from build123d import *

# Parameters (mm, degrees)
SKETCH3_R           = 15
BOSS_EXTRUDE1_DEPTH = 20
SKETCH4_R           = 2.5
CUT_EXTRUDE1_DEPTH  = 30.154759474
CUT_EXTRUDE2_DEPTH  = 4.5
SKETCH7_W           = 9
SKETCH7_H           = 4.5
CUT_EXTRUDE3_DEPTH  = 30.154759474
BOSS_EXTRUDE3_DEPTH = 10
SKETCH9_R           = 2.5
CUT_EXTRUDE4_DEPTH  = 30
SKETCH12_R          = 23.5
BOSS_EXTRUDE6_DEPTH = 75
SKETCH13_R          = 19
CUT_EXTRUDE6_DEPTH  = 143.195288401
SKETCH14_R          = 19
BOSS_EXTRUDE7_DEPTH = 5
SKETCH15_R          = 1.5
SKETCH15_R_2        = 2.5
CUT_EXTRUDE8_DEPTH  = 5


with BuildPart() as part:
    # Sketch3 → Boss-Extrude1 (new body)
    with BuildSketch(Plane(origin=(0, 0, 0), x_dir=(1, 0, 0), z_dir=(0, 1, 0))):
        with Locations(Location((0, 0, 0), (0, 0, 270))):
            Circle(SKETCH3_R)
    extrude(amount=-BOSS_EXTRUDE1_DEPTH)

    # Sketch4 → Cut-Extrude1 (cut, through all)
    with BuildSketch(Plane(origin=(0, 0, 0), x_dir=(1, 0, 0), z_dir=(0, 1, 0))):
        with Locations(Location((0, 0, 0), (0, 0, 270))):
            Circle(SKETCH4_R)
    extrude(amount=-CUT_EXTRUDE1_DEPTH, mode=Mode.SUBTRACT)

    # Sketch6 → Cut-Extrude2 (cut)
    with BuildSketch(Plane(origin=(0, -5, 0), x_dir=(1, 0, 0), z_dir=(0, 1, 0))):
        Polygon((4.5, -2.598076211), (4.5, 2.598076211), (0, 5.196152423), (-4.5, 2.598076211), (-4.5, -2.598076211), (0, -5.196152423), align=None)
    extrude(amount=-CUT_EXTRUDE2_DEPTH, mode=Mode.SUBTRACT)

    # Sketch7 → Cut-Extrude3 (cut, through all)
    with BuildSketch(Plane.XY):
        with Locations((0, -7.25)):
            Rectangle(SKETCH7_W, SKETCH7_H)
    extrude(amount=CUT_EXTRUDE3_DEPTH, mode=Mode.SUBTRACT)

    # Sketch8 → Boss-Extrude3 (add, symmetric)
    with BuildSketch(Plane(origin=(0, 0, 0), x_dir=(0, 0, -1), z_dir=(1, 0, 0))):
        with BuildLine():
            Line((0, 0), (0, -20))
            add(Edge.make_bspline(
                [(0, -20), (27.284263103, -24.07033424), (42.456200025, -63.400009775), (20, -80)],
                knots=[0, 0, 0, 0, 1, 1, 1, 1], degree=3))
            Line((20, -80), (67.5, -80))
            add(Edge.make_bspline(
                [(0, 0), (41.415251378, -8.894775063), (64.240572417, -43.774170089), (67.5, -80)],
                knots=[0, 0, 0, 0, 1, 1, 1, 1], degree=3))
        make_face()
    extrude(amount=BOSS_EXTRUDE3_DEPTH, both=True)

    # Sketch9 → Cut-Extrude4 (cut)
    with BuildSketch(Plane(origin=(0, 0, 0), x_dir=(1, 0, 0), z_dir=(0, 1, 0))):
        with Locations(Location((0, 0, 0), (0, 0, 270))):
            Circle(SKETCH9_R)
    extrude(amount=-CUT_EXTRUDE4_DEPTH, mode=Mode.SUBTRACT)

    # Sketch12 → Boss-Extrude6 (add)
    with BuildSketch(Plane.XY.offset(-10)):
        with Locations((0, -95)):
            Circle(SKETCH12_R)
    extrude(amount=-BOSS_EXTRUDE6_DEPTH)

    # Sketch13 → Cut-Extrude6 (cut, through all)
    with BuildSketch(Plane.XY.offset(-10)):
        with Locations((0, -95)):
            Circle(SKETCH13_R)
    extrude(amount=-CUT_EXTRUDE6_DEPTH, mode=Mode.SUBTRACT)

    # Sketch14 → Boss-Extrude7 (add)
    with BuildSketch(Plane.XY.offset(-10)):
        with Locations((0, -95)):
            Circle(SKETCH14_R)
    extrude(amount=-BOSS_EXTRUDE7_DEPTH)

    # Sketch15 → Cut-Extrude8 (cut)
    with BuildSketch(Plane.XY.offset(-10)):
        with Locations((15.9, -95)):
            Circle(SKETCH15_R)
        with Locations((7.95, -108.76980392)):
            Circle(SKETCH15_R)
        with Locations((-7.95, -108.76980392)):
            Circle(SKETCH15_R)
        with Locations((-15.9, -95)):
            Circle(SKETCH15_R)
        with Locations((-7.95, -81.23019608)):
            Circle(SKETCH15_R)
        with Locations((7.95, -81.23019608)):
            Circle(SKETCH15_R)
        with Locations((0, -104.5)):
            Circle(SKETCH15_R_2)
    extrude(amount=-CUT_EXTRUDE8_DEPTH, mode=Mode.SUBTRACT)


solid = part.part
The listing builds one solid part. Answer for the finished solid, in the listing's coordinates (mm). A direction names the side the tool comes from. Coordinates: 2 decimals unless noted, no trailing zeros. Order: outer loops, then holes, each group sorted by start corner. A loop starts at its lowest first (then second) coordinate and runs counter-clockwise, first axis right, second up.
Q1. A cutting plane is placed at A-A, the plane x = 12. Write down the section's boundary in (y, z), and give its area (3 significant figures).
Q2. A cutting plane is placed at C-C, the plane z = -74.5. Write down the section's boundary in (x, y), and give its area (3 significant figures).
Q3. Which of the six approach directions +Z, -Z, +X, -X, +Y, -Y give full straight-line access (tool end or side, diameter ignored) to faces 4 (the face through (4.506, -9.86, 14.307)), 5 (the face through (0, -95, -15)), 6 (the face through (-4.5, -7, 7)), 7 (the face through (7.625, -110.234, -12.465))?
Q4. Consider line 1 (Y direction, x = 3, z = 5); line 2 (X direction, y = -82, z = -11.5); line 3 (Y direction, x = 7, z = -12). Determine where each line is inside the solid, lowest interval first.
Q5. Given P1, Ø3.5, axis at x = -7.95, y = -81.23, coming from the +Z side; P2, Ø5, axis at y = -6.5, z = 3.5, coming from the -X side; P3, Ø21, axis at x = -3, z = 6.5, coming from the -Y side; P4, Ø1.8, axis at x = 15.9, y = -95, coming from the -Z side, each flat-ended and moving along its own axis, determine where each tip first touches the part or whether it passes through.
Q6. A cutting plane is placed at B-B, the plane z = 4.5. Write down the section's boundary in (x, y).
Q7. For a pull along Z with two mould halves and no side action, classify faces 1 (the face through (-0.33, -10.1, -2.48)), 2 (the face through (9, -112, -85)), 3 (the face through (0, -5, 7)) as pulls with the +Z half, pulls with the -Z half, needs draft (parallel to the pull), parting line crosses it, or undercut.
Answers follow:
1. outline: (-115.21, -85) - (-109.73, -85) - (-109.73, -15) - (-80.27, -15) - (-80.27, -85) - (-74.79, -85) - (-74.79, -10) - (-115.21, -10) - close; (-20, -9) - (0, -9) - (0, 9) - (-20, 9) - close
1. area: 1,330 mm2
2. outline: circle Ø47 at (0, -95); hole circle Ø38 at (0, -95)
2. area: 601 mm2
3. face 4: +Y
3. face 5: -Z
3. face 6: +Z
3. face 7: +Z, -Z
4. line 1: y = -20 to -9.5, -5 to 0
4. line 2: x = -19.58 to -9.24, -6.66 to 6.66, 9.24 to 19.58
4. line 3: y = -117.43 to -109.93, -107.61 to -82.39, -80.07 to -72.57, -24.39 to 0
5. P1: stops at z = -10
5. P2: stops at x = -14.97
5. P3: stops at y = -20.87
5. P4: passes through
6. outline: (-14.31, -20) - (14.31, -20) - (14.31, 0) - (-14.31, 0) - close; hole (-4.5, -9.5) - (4.5, -9.5) - (4.5, -5) - (-4.5, -5) - close
7. face 1: undercut
7. face 2: pulls with the -Z half
7. face 3: needs draft
